Geometry: final body of the model. Coordinates: model frame, mm. A direction names the side the tool comes from. Coordinates: 2 decimals unless noted, no trailing zeros. Order: outer loops, then holes, each group sorted by start corner. A loop starts at its lowest first (then second) coordinate and runs counter-clockwise, first axis right, second up. Notation, with made-up numbers: (76.5, -35.75) -> (129.5, -35.75) arc R19 ccw to (129.5, -2.75) -> close; hole circle Ø4 at (27.25, -4.75). An arc over 180 degrees is marked (long way). Answer in a Markdown table with one row per item. Add a question column.
1) Pull-direction query (X, two-part tool) for faces 5 (the face through (70.047, -2, 3)), 6 (the face through (-88.9, 0, -3)), 7 (the face through (73.82, -9.36, 26.35)); classes: +X half, -X half, draft (parallel to the pull), parting line (faces both ways), or undercut.
2) Ray query, line 1 (Y direction, x = -40, z = 31); line 2 (X direction, y = -1, z = 34); line 3 (X direction, y = -10.5, z = 2.5). Return the intervals inside material, ascending. Write a range as from..to.
3) Set-up query: faces 1 (the face through (-73.821, 9.918, 25.416)), 2 (the face through (74, -16, 6.059)), 3 (the face through (-69.171, -2, 3)), 4 (the face through (-74, -16, 6.059)). Return all of +Z, -Z, +X, -X, +Y, -Y with unobstructed straight access to the full face (end or side cutting, diameter ignored); none if empty.
4) Contact query for flat-ended pins moving along their axis: P1, Ø1, axis at x = -58.5, y = 2.5, coming from the +Z side; P2, Ø0.7, axis at y = -0.5, z = 6, coming from the -X side; P3, Ø5, axis at y = -2.5, z = 36, coming from the -X side. Output: stop coordinate, or through.
5) Section query B-B on z = 3. Return the cut outline in (x, y).
6) Section query A-A on x = 9.5. Return the cut outline in (y, z).
7) Section query D-D on y = 5.5. Return the cut outline in (x, z), then the cut area to 3 significant figures.
8) Section query C-C on z = 12. Return the cut outline in (x, y), then the cut area to 3 significant figures.
```python
from build123d import *

# Parameters (mm, degrees)
F0_W      = 177.8
F0_H      = 38.1
F1_DEPTH  = 5.588
F4_DEPTH  = 4.826
F6_DEPTH  = 11.43
F8_DEPTH  = 233.426
F11_DEPTH = 38.1
F13_W     = 139.2178796232
F13_H     = 23.7698024139
F14_DEPTH = 51.308


with BuildPart() as f1:
    # F0 (on Top) → F1 (new body)
    with BuildSketch(Plane.XY):
        Rectangle(F0_W, F0_H)
    extrude(amount=F1_DEPTH)

    # F3 (on offset) → F4 (join)
    with BuildSketch(Plane.YZ.offset(76.2)):
        Polygon((0, 46.0882298648), (-18.9831927419, 6.0590645298), (-13.1481755525, 6.0590645298), (0, 34.8115004599), (13.6455185711, 5.3136325441), (19.5630453527, 5.3136325441), align=None)
    extrude(amount=-F4_DEPTH)

    # F5: F1 across plane


with BuildPart() as f1_1:
    add(f1.part)
    add(f1.part.mirror(Plane.YZ))

    # F6 (add): a face of the model
    f6_faces = [f1_1.faces().sort_by_distance(p)[0] for p in [
        (0, 0, 0),
    ]]
    extrude(f6_faces, amount=F6_DEPTH)

    # F7 (on face) → F8 (cut)
    with BuildSketch(Plane.XZ.offset(19.05)):
        with BuildLine():
            Line((-55.2403405309, -11.43), (52.1429181099, -11.43))
            ThreePointArc((52.1429181099, -11.43), (-1.5487112105, -3.1079738738), (-55.2403405309, -11.43))
        make_face()
    extrude(amount=-F8_DEPTH, mode=Mode.SUBTRACT)

    # F10 (on offset) → F11 (join)
    with BuildSketch(Plane.XZ.offset(19.05)):
        with BuildLine():
            Line((-71.5217785408, 5.7395980693), (71.2262214592, 5.7395980693))
            ThreePointArc((71.2262214592, 5.7395980693), (-0.1477785408, 40.3939508929), (-71.5217785408, 5.7395980693))
        make_face()
    extrude(amount=-F11_DEPTH)

    # F13 (on offset) → F14 (cut)
    with BuildSketch(Plane.XY.offset(50.8254)):
        with Locations((0.4383567721, -1.7096721567)):
            Rectangle(F13_W, F13_H)
    extrude(amount=-F14_DEPTH, mode=Mode.SUBTRACT)


solid = f1_1.part
```
Result:
| question | item | result |
|---|---|---|
| 1 | face 5 | undercut |
| 1 | face 6 | -X half |
| 1 | face 7 | draft |
| 2 | line 1 | -19.05..-13.59, 10.18..19.05 |
| 2 | line 2 | -76.2..-71.37, 71.37..76.2 |
| 2 | line 3 | -88.9..-69.17, 70.05..88.9 |
| 3 | face 1 | +Z, -X, +Y |
| 3 | face 2 | +X, -Y |
| 3 | face 3 | +Z |
| 3 | face 4 | -X, -Y |
| 4 | P1 | z = -0.48 |
| 4 | P2 | x = -71.52 |
| 4 | P3 | x = -76.2 |
| 5 | outline | (-88.9, -19.05) -> (88.9, -19.05) -> (88.9, 19.05) -> (-88.9, 19.05) -> close; hole (-69.17, -13.59) -> (70.05, -13.59) -> (70.05, 10.18) -> (-69.17, 10.18) -> close |
| 6 | outline | (-19.05, -3.45) -> (19.05, -3.45) -> (19.05, 5.59) -> (10.18, 5.59) -> (10.18, -0.48) -> (-13.59, -0.48) -> (-13.59, 5.59) -> (-19.05, 5.59) -> close; (-19.05, 5.74) -> (-13.59, 5.74) -> (-13.59, 39.88) -> (-19.05, 39.88) -> close; (10.18, 5.74) -> (19.05, 5.74) -> (19.05, 39.88) -> (10.18, 39.88) -> close |
| 7 | outline | (-88.9, -11.43) -> (-55.24, -11.43) arc R177.36 cw to (52.14, -11.43) -> (88.9, -11.43) -> (88.9, 5.59) -> (70.05, 5.59) -> (70.05, -0.48) -> (-69.17, -0.48) -> (-69.17, 5.59) -> (-88.9, 5.59) -> close; (-76.2, 22.92) -> (-71.37, 22.92) -> (-71.37, 34.62) -> (-76.2, 34.62) -> close; (-71.52, 5.74) -> (-69.17, 5.74) -> (-69.17, 8.6) arc R90.83 ccw to start; (70.05, 5.74) -> (71.23, 5.74) arc R90.83 ccw to (70.05, 7.21) -> close; (71.37, 22.92) -> (76.2, 22.92) -> (76.2, 34.62) -> (71.37, 34.62) -> close |
| 7 | area | 1,700 mm2 |
| 8 | outline | (-76.2, -16.17) -> (-71.37, -16.17) -> (-71.37, -10.43) -> (-76.2, -10.43) -> close; (-76.2, 10.55) -> (-71.37, 10.55) -> (-71.37, 16.36) -> (-76.2, 16.36) -> close; (-66.12, -19.05) -> (65.82, -19.05) -> (65.82, -13.59) -> (-66.12, -13.59) -> close; (-66.12, 10.18) -> (65.82, 10.18) -> (65.82, 19.05) -> (-66.12, 19.05) -> close; (71.37, -16.17) -> (76.2, -16.17) -> (76.2, -10.43) -> (71.37, -10.43) -> close; (71.37, 10.55) -> (76.2, 10.55) -> (76.2, 16.36) -> (71.37, 16.36) -> close |
| 8 | area | 2,000 mm2 |
